Could you check a few things on this model? Use its own coordinates, in mm. A direction names the side the tool comes from. Give positions to 0.01 mm unless a question says otherwise; leave off trailing zeros. Order: outer loops, then holes, each group sorted by start corner. A loop starts at its lowest first (then second) coordinate and runs counter-clockwise, first axis right, second up.
from build123d import *

# Parameters (mm, degrees)
SKIZZE1_R                       = 1.6
AUFSATZ_LINEAR_AUSTRAGEN1_DEPTH = 5


with BuildPart() as part:
    # Skizze1 → Aufsatz-Linear austragen1 (new body)
    with BuildSketch(Plane.XY):
        Polygon((35, 250), (45, 250), (45, 255), (55, 255), (55, 250), (65, 250), (65, 255), (75, 255), (75, 250), (85, 250), (85, 255), (95, 255), (95, 250), (105, 250), (105, 255), (115, 255), (115, 250), (125, 250), (125, 255), (135, 255), (135, 250), (145, 250), (145, 255), (155, 255), (155, 250), (165, 250), (165, 255), (175, 255), (175, 250), (185, 250), (185, 255), (195, 255), (195, 250), (205, 250), (205, 255), (215, 255), (215, 250), (225, 250), (255, 220), (260, 220), (260, 210), (255, 210), (255, 200), (260, 200), (260, 190), (255, 190), (255, 180), (260, 180), (260, 170), (255, 170), (255, 160), (260, 160), (260, 150), (255, 150), (255, 140), (260, 140), (260, 130), (255, 130), (255, 120), (260, 120), (260, 110), (255, 110), (255, 100), (260, 100), (260, 90), (255, 90), (255, 80), (260, 80), (260, 70), (255, 70), (255, 60), (260, 60), (260, 50), (255, 50), (255, 40), (260, 40), (260, 30), (255, 30), (255, 20), (260, 20), (260, 10), (255, 10), (255, 0), (5, 0), (5, 10), (0, 10), (0, 20), (5, 20), (5, 30), (0, 30), (0, 40), (5, 40), (5, 50), (0, 50), (0, 60), (5, 60), (5, 70), (0, 70), (0, 80), (5, 80), (5, 90), (0, 90), (0, 100), (5, 100), (5, 110), (0, 110), (0, 120), (5, 120), (5, 130), (0, 130), (0, 140), (5, 140), (5, 150), (0, 150), (0, 160), (5, 160), (5, 170), (0, 170), (0, 180), (5, 180), (5, 190), (0, 190), (0, 200), (5, 200), (5, 210), (0, 210), (0, 220), (5, 220), align=None)
        with Locations((20, 215)):
            Circle(SKIZZE1_R, mode=Mode.SUBTRACT)
        with Locations((30, 215)):
            Circle(SKIZZE1_R, mode=Mode.SUBTRACT)
        with Locations((240, 215)):
            Circle(SKIZZE1_R, mode=Mode.SUBTRACT)
        with Locations((230, 215)):
            Circle(SKIZZE1_R, mode=Mode.SUBTRACT)
        Polygon((65, 218.971165398), (195, 218.971165398), (225, 188.971165398), (225, 78.971165398), (35, 78.971165398), (35, 188.971165398), align=None, mode=Mode.SUBTRACT)
    extrude(amount=AUFSATZ_LINEAR_AUSTRAGEN1_DEPTH)


solid = part.part
Item 1: Imagine slicing it at A-A on x = 121.5. List the corners of the cut face in (y, z) for me.
Findings:
outline: (0, 0) - (78.97, 0) - (78.97, 5) - (0, 5) - close; (218.97, 0) - (250, 0) - (250, 5) - (218.97, 5) - close
Item 2: We'd pull the mould along X, two halves only. Please class faces 1 (the flat face through (240, 235, 2)), 2 (the flat face through (132, 73, 5)), 3 (the flat face through (209.79, 204.18, 2.46)): +X half, -X half, draft (parallel to the pull), parting line (faces both ways), or undercut.
Findings:
face 1: +X half
face 2: draft
face 3: undercut
Item 3: Imagine slicing it at C-C on z = 1.05. Give the number of separate pieces and of enclosed holes in the cut face, then the cut area to 3 significant figures.
Findings:
separate pieces: 1
enclosed holes: 5
area: 37,400 mm2
Item 4: For pin 1 (1.5 mm diameter, centred on x = 99.5, z = 1.5, fed in from +Y); pin 2 (2.5 mm diameter, centred on x = 257.5, z = 3, fed in from +Y); pin 3 (2.5 mm diameter, centred on x = 3.5, z = 2.5, fed in from -Y), each with a flat end and sliding along its axis, tell me the tip position at first contact or that it passes through.
Findings:
pin 1: stops at y = 250
pin 2: stops at y = 220
pin 3: stops at y = 10
Item 5: Imagine slicing it at B-B on y = 203. List the corners of the cut face in (x, z) for me.
Findings:
outline: (5, 0) - (49.03, 0) - (49.03, 5) - (5, 5) - close; (210.97, 0) - (255, 0) - (255, 5) - (210.97, 5) - close
Item 6: Please list where these lines run through material, in increasing order: line 1 along X through (y, z) = (215, 2.1); line 2 along X through (y, z) = (184, 1.05); line 3 along X through (y, z) = (151, 2.45).
Findings:
line 1: x = 0 to 18.4, 21.6 to 28.4, 31.6 to 61.03, 198.97 to 228.4, 231.6 to 238.4, 241.6 to 260
line 2: x = 5 to 35, 225 to 255
line 3: x = 0 to 35, 225 to 260
Item 7: For faces 4 (the flat face through (132, 73, 0)), 5 (the flat face through (49.79, 203.76, 2.46)), which set-ups out of +Z, -Z, +X, -X, +Y, -Y let a thin tool reach every point of the face, with its end or its side?
Findings:
face 4: -Z, +X, -X, +Y, -Y
face 5: +Z, -Z
